Can you work these out from the model? Positions are in its coordinate system, mm. A direction names the side the tool comes from. Give positions to 0.01 mm unless a question says otherwise; leave off trailing zeros. Order: outer loops, then holes, each group sorted by start corner. A loop starts at its lowest first (then second) coordinate and runs counter-clockwise, first axis right, second up. Notation, with made-up numbers: M 6.5,-2 L 33.5,-2 A27 ccw 33.5,36 Z; hole C 86.5,-28 d7. An arc over 180 degrees is marked long. Answer as a JSON object with one key per item and string values.
```python
from build123d import *

# Parameters (mm, degrees)
SKETCH1_R           = 86.6
BOSS_EXTRUDE1_DEPTH = 50
SKETCH2_R           = 6
CUT_EXTRUDE1_DEPTH  = 50
SKETCH3_W           = 8.5
SKETCH3_H           = 8
SKETCH3_W_2         = 72
SKETCH3_H_2         = 30
CUT_EXTRUDE2_DEPTH  = 27
FILLET1_R           = 5
FILLET2_R           = 5
CUT_EXTRUDE3_START  = -32
SKETCH4_R           = 4
CUT_EXTRUDE3_DEPTH  = 32
SKETCH5_R           = 5.042988513
CUT_EXTRUDE4_DEPTH  = 4


with BuildPart() as part:
    # Sketch1 → Boss-Extrude1 (new body)
    with BuildSketch(Plane(origin=(0, 0, 0), x_dir=(1, 0, 0), z_dir=(0, 1, 0))):
        with Locations(Location((0, 0, 0), (0, 0, 270))):
            Circle(SKETCH1_R)
    extrude(amount=BOSS_EXTRUDE1_DEPTH)

    # Sketch2 → Cut-Extrude1 (cut)
    with BuildSketch(Plane(origin=(0, 50, 0), x_dir=(1, 0, 0), z_dir=(0, 1, 0))):
        with Locations(Location((0, 50, 0), (0, 0, 270))):
            Circle(SKETCH2_R)
        with Locations(Location((35.355339059, 35.355339059, 0), (0, 0, 270))):
            Circle(SKETCH2_R)
        with Locations(Location((35.355339059, -35.355339059, 0), (0, 0, 270))):
            Circle(SKETCH2_R)
        with Locations(Location((-35.355339059, -35.355339059, 0), (0, 0, 270))):
            Circle(SKETCH2_R)
        with Locations(Location((-50, 0, 0), (0, 0, 270))):
            Circle(SKETCH2_R)
        with Locations(Location((-35.355339059, 35.355339059, 0), (0, 0, 270))):
            Circle(SKETCH2_R)
    extrude(amount=-CUT_EXTRUDE1_DEPTH, mode=Mode.SUBTRACT)

    # Sketch3 → Cut-Extrude2 (cut)
    with BuildSketch(Plane(origin=(0, 50, 0), x_dir=(1, 0, 0), z_dir=(0, 1, 0))):
        with Locations((4.25, -19)):
            Rectangle(SKETCH3_W, SKETCH3_H)
        with Locations((-4.25, -19)):
            Rectangle(SKETCH3_W, SKETCH3_H)
        Rectangle(SKETCH3_W_2, SKETCH3_H_2)
    extrude(amount=-CUT_EXTRUDE2_DEPTH, mode=Mode.SUBTRACT)

    # Fillet1
    fillet1_edges = [part.edges().sort_by_distance(p)[0] for p in [
        (0, 23, -15),
    ]]
    fillet(fillet1_edges, radius=FILLET1_R)

    # Fillet2
    fillet2_edges = [part.edges().sort_by_distance(p)[0] for p in [
        (-22.25, 23, 15),
        (22.25, 23, 15),
    ]]
    fillet(fillet2_edges, radius=FILLET2_R)

    # Sketch4 → Cut-Extrude3 (cut)
    with BuildSketch(Plane(origin=(0, 50, 0), x_dir=(1, 0, 0), z_dir=(0, 1, 0)).offset(CUT_EXTRUDE3_START)):
        with BuildLine():
            Line((86.507571923, 4), (36, 4))
            Line((36, 4), (36, -4))
            Line((36, -4), (86.507571923, -4))
            ThreePointArc((86.507571923, -4), (86.576889897, -2.000533863), (86.6, 0))
            ThreePointArc((86.6, 0), (86.576889897, 2.000533863), (86.507571923, 4))
        make_face()
        with BuildLine():
            Line((36, 4), (18.507571923, 4))
            ThreePointArc((18.507571923, 4), (21.335999048, 2.828427125), (22.507571923, 0))
            ThreePointArc((22.507571923, 0), (21.335999048, -2.828427125), (18.507571923, -4))
            Line((18.507571923, -4), (36, -4))
            Line((36, -4), (36, 4))
        make_face()
        with Locations((18.507571923, 0)):
            Circle(SKETCH4_R)
        with BuildLine():
            ThreePointArc((86.507571923, -4), (90.507571923, 0), (86.507571923, 4))
            ThreePointArc((86.507571923, 4), (86.576889897, 2.000533863), (86.6, 0))
            ThreePointArc((86.6, 0), (86.576889897, -2.000533863), (86.507571923, -4))
        make_face()
    extrude(amount=CUT_EXTRUDE3_DEPTH, mode=Mode.SUBTRACT)

    # Sketch5 → Cut-Extrude4 (cut)
    with BuildSketch(Plane(origin=(0, 50, 0), x_dir=(1, 0, 0), z_dir=(0, 1, 0))):
        with Locations(Location((-16, -23, 0), (0, 0, 270))):
            Circle(SKETCH5_R)
        with Locations(Location((16, -23, 0), (0, 0, 270))):
            Circle(SKETCH5_R)
        with Locations(Location((16, 23, 0), (0, 0, 270))):
            Circle(SKETCH5_R)
        with Locations(Location((-16, 23, 0), (0, 0, 270))):
            Circle(SKETCH5_R)
    extrude(amount=-CUT_EXTRUDE4_DEPTH, mode=Mode.SUBTRACT)


solid = part.part
```
1) I want a section at C-C on y = 33. Write out the boundary of the cut face in (x, z).
Results found:
{"outline": "M -36,-15 L -36,15 L -8.5,15 L -8.5,23 L 8.5,23 L 8.5,15 L 36,15 L 36,4 L 86.51,4 A86.6 ccw long 86.51,-4 L 36,-4 L 36,-15 Z; hole C -50,0 d12; hole C -35.36,-35.36 d12; hole C -35.36,35.36 d12; hole C 0,-50 d12; hole C 35.36,-35.36 d12; hole C 35.36,35.36 d12"}
2) I want a section at D-D on x = 39. Write out the boundary of the cut face in (y, z), and give its area (3 significant figures).
Results found:
{"outline": "M 0,-77.32 L 50,-77.32 L 50,-40.12 L 0,-40.12 Z; M 0,-30.59 L 50,-30.59 L 50,-4 L 18,-4 L 18,4 L 50,4 L 50,30.59 L 0,30.59 Z; M 0,40.12 L 50,40.12 L 50,77.32 L 0,77.32 Z", "area": "6,520 mm²"}
3) I want a section at A-A on z = 0. Write out the boundary of the cut face in (x, y).
Results found:
{"outline": "M -86.6,0 L -56,0 L -56,50 L -86.6,50 Z; M -44,0 L 86.6,0 L 86.6,18 L 14.51,18 L 14.51,23 L -36,23 L -36,50 L -44,50 Z"}
4) For faces 3 (the face through (19.408, 48.028, 19.283)), 4 (the face through (29.5, 25.35, -36.66)), 5 (the face through (60, 34, 4)), which set-ups out of +Z, -Z, +X, -X, +Y, -Y let a thin tool reach every point of the face, with its end or its side?
Results found:
{"face 3": "+Y", "face 4": "+Y, -Y", "face 5": "+X, +Y"}
5) I'm going to push flat-ended pins straight in: pin 1 Ø3 at (x, z) = (16, -24) entering from +Y; pin 2 Ø6 at (y, z) = (43, 38.5) entering from +X; pin 3 Ø10 at (y, z) = (19, 45.5) entering from +X; pin 4 Ø1 at (x, z) = (52, -58.5) entering from -Y. Where does each tip first touch, or does it pass through?
Results found:
{"pin 1": "stops at y = 46", "pin 2": "stops at x = 78.99", "pin 3": "stops at x = 76.55", "pin 4": "stops at y = 0"}
6) Thinking about a two-plate mould opening in X: for faces 1 (the face through (50, 18, 0)), 2 (the face through (29.5, 25.35, 34.05)), which applies, pulls with the +X half, pulls with the -X half, needs draft (parallel to the pull), parting line crosses it, or undercut?
Results found:
{"face 1": "needs draft", "face 2": "undercut"}
7) I want a section at B-B on x = 0. Write out the boundary of the cut face in (y, z), and give its area (3 significant figures).
Results found:
{"outline": "M 0,-86.6 L 50,-86.6 L 50,-56 L 0,-56 Z; M 0,-44 L 50,-44 L 50,-15 L 28,-15 A5 cw 23,-10 L 23,23 L 50,23 L 50,86.6 L 0,86.6 Z", "area": "7,040 mm²"}
8) I need wall thicknesses on L1, parallel to Z at x = -19, y = 47.5; L2, parallel to Z at x = 38, y = 9; L3, parallel to X at y = 6, z = -31. Which ranges of each line are inside material? Lowest first, please.
Results found:
{"L1": "z = -84.49 to -27.05, -18.95 to -15, 15 to 18.95, 27.05 to 84.49", "L2": "z = -77.82 to -40.74, -29.97 to 29.97, 40.74 to 77.82", "L3": "x = -80.86 to -39.48, -31.23 to 31.23, 39.48 to 80.86"}
